```python
from build123d import *

# Parameters (mm, degrees)
BOSS_EXTRUDE1_DEPTH = 5.08
SKETCH2_R           = 1.27
CUT_EXTRUDE1_DEPTH  = 10


with BuildPart() as part:
    # Sketch1 → Boss-Extrude1 (new body)
    with BuildSketch(Plane(origin=(0, 0, 0), x_dir=(0, 0, -1), z_dir=(1, 0, 0))):
        with BuildLine():
            Line((-30.090800845, -0.203985657), (-18.085491541, -29.008366119))
            Line((-18.085491541, -29.008366119), (19.045846251, -18.010521201))
            Line((19.045846251, -18.010521201), (30.090800845, -3.045918822))
            Line((30.090800845, -3.045918822), (30.090800845, 19.650147268))
            add(Edge.make_bspline(
                [(30.090800845, 19.650147268), (28.037602076, 22.726688549), (23.033153586, 26.860701903), (14.987767723, 29.008366119), (7.524677055, 28.774184664), (0.603908496, 27.036559666), (-6.727735861, 23.899909345), (-13.041122451, 19.375109172), (-21.198561263, 11.380500033), (-26.40610074, 4.431018315), (-30.090800845, -0.203985657)],
                knots=[0, 0, 0, 0, 0.148846654, 0.252987858, 0.329376305, 0.448668947, 0.539169161, 0.650373484, 0.760197294, 1, 1, 1, 1], degree=3))
        make_face()
    extrude(amount=BOSS_EXTRUDE1_DEPTH)

    # Sketch2 → Cut-Extrude1 (cut)
    with BuildSketch(Plane(origin=(5.08, 0, 0), x_dir=(0, 0, -1), z_dir=(1, 0, 0))):
        with Locations((-27.1490755, -0.589985571)):
            Circle(SKETCH2_R)
        with Locations((-16.665824451, -25.950337288)):
            Circle(SKETCH2_R)
        with Locations((17.412184036, -15.937519564)):
            Circle(SKETCH2_R)
        with Locations((27.54487652, -2.200233664)):
            Circle(SKETCH2_R)
        with Locations((27.54487652, 19.042163131)):
            Circle(SKETCH2_R)
        with Locations((1.198662119, 24.319887944)):
            Circle(SKETCH2_R)
    extrude(amount=-CUT_EXTRUDE1_DEPTH, mode=Mode.SUBTRACT)


solid = part.part
```
CAD build for the part. Positions are in the model's coordinates, mm. Round coordinates to 2 decimals unless told otherwise and drop trailing zeros. Write each loop counter-clockwise with the first axis right and the second up, starting at its lowest first coordinate (ties: lowest second). Pieces come first, ordered by that corner, then holes. Notation, with made-up numbers: (41, 63) - (57, 63) arc R27 ccw to (57, 98) - close; hole circle Ø11 at (-17.75, -13.5). An arc over 180 degrees is marked (long way). Write item = value, one per line. Start each with the question number.
Q1. Probe L1, parallel to Y at x = 1.85, z = -17; L2, parallel to Z at x = 1.1, y = 9.5; L3, parallel to Z at x = 1.9, y = -15.5. List the from-to ranges inside material, lowest first. Write a range as from..to.
Q2. Drop flat-ended pins along their axis: pin 1 (1 mm diameter, centred on x = 2, z = -3.5, fed in from -Y); pin 2 (3 mm diameter, centred on x = 2, z = 18, fed in from +Y); pin 3 (3 mm diameter, centred on x = 1.5, y = -9, fed in from +Z). Give the stop position or say it passes through.
Q3. Band-saw the part on B-B (y = -8). Give the cut face in (x, z), then the cut area to 3 significant figures.
Q4. Mould opens along Z. For faces 1 (the flat face through (3, 8, -30.091)), 2 (the flat face through (5.08, 0, 0)), 3 (the cylindrical face through (2.58, 25.58, -1.03)) say: pulls with the +Z half, pulls with the -Z half, needs draft (parallel to the pull), parting line crosses it, or undercut.
Q5. Band-saw the part on A-A (x = 3.5). Count the separate pieces of the cut face and the enclosed holes in it, then the cut area to 3 significant figures.
Answers below:
q1.L1 = -18.62..-17.14, -14.74..28.33
q1.L2 = -30.09..22.35
q1.L3 = -20.9..-18.6, -16.22..23.72
q2.pin_1 = -22.76
q2.pin_2 = 15.93
q2.pin_3 = 27.05
q3.outline = (0, -26.43) - (5.08, -26.43) - (5.08, 26.84) - (0, 26.84) - close
q3.area = 271 mm2
q4.face_1 = pulls with the -Z half
q4.face_2 = needs draft
q4.face_3 = undercut
q5.separate_pieces = 1
q5.enclosed_holes = 6
q5.area = 2,420 mm2
